Can you work these out from the model? Positions are in its coordinate system, mm. Face numbers are marked on the shaded views. Give positions to 0.01 mm unless a question says otherwise; leave off trailing zeros. Write each loop counter-clockwise with the first axis right and the second up, starting at its lowest first coordinate (ties: lowest second). Pieces come first, ordered by that corner, then holes. Notation, with made-up numbers: (20.5, 27) -> (51.5, 27) arc R29 ccw to (51.5, 64) -> close; hole circle Ø11 at (-35.75, 60). An arc over 180 degrees is marked (long way). Answer as CSV lines item,"result". Start each with the question number.
1. If we section it at D-D on y = -1.65: Write out the boundary of the cut face in (x, z).
2. I need wall thicknesses on line 1 (Y direction, x = 11.5, z = 3.25); line 2 (X direction, y = -0.9, z = 3.2); line 3 (X direction, y = -0.15, z = 2.35). Which ranges of each line are inside material? Lowest first, please. Write a range as [from, to].
3. If we section it at B-B on y = -0.6: Write out the boundary of the cut face in (x, z).
4. If we section it at A-A on z = 3.5: Count the separate pieces of the cut face and the enclosed holes in it, plus the area to 3 significant figures.
5. If we section it at C-C on y = 0.55: Write out the boundary of the cut face in (x, z).
6. If we mould it in two halves opening along Y, with no side actions, what happens to the marked faces 1, 2 and 3? For each: pulls with the +Y half, pulls with the -Y half, needs draft (parallel to the pull), parting line crosses it, or undercut.
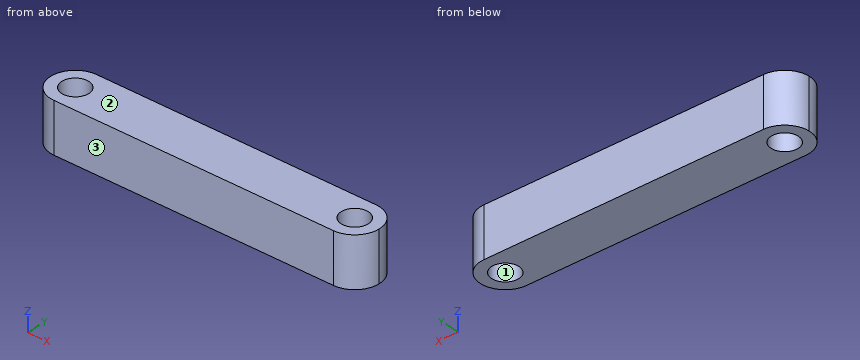
```python
from build123d import *

# Parameters (mm, degrees)
SKETCH_1_W          = 27
SKETCH_1_H          = 4
EXTRUDE_1_DEPTH     = 4
FILLET_1_R          = 2
SKETCH_2_R          = 1.1
CUT_EXTRUDE_1_DEPTH = 13


with BuildPart() as part:
    # 草图1 → 凸台-拉伸1 (new body)
    with BuildSketch(Plane.XY):
        Rectangle(SKETCH_1_W, SKETCH_1_H)
    extrude(amount=EXTRUDE_1_DEPTH)

    # 圆角1
    fillet_1_edges = [part.edges().sort_by_distance(p)[0] for p in [
        (-13.5, -2, 2),
        (-13.5, 2, 2),
        (13.5, -2, 2),
        (13.5, 2, 2),
    ]]
    fillet(fillet_1_edges, radius=FILLET_1_R - 0.0001)  # a hair under: the kernel refuses the full size

    # 草图2 → 切除-拉伸1 (cut)
    with BuildSketch(Plane.XY.offset(4)):
        with Locations((-11.5, 0)):
            Circle(SKETCH_2_R)
        with Locations((11.5, 0)):
            Circle(SKETCH_2_R)
    extrude(amount=-CUT_EXTRUDE_1_DEPTH, mode=Mode.SUBTRACT)


solid = part.part
```
Computed values:
1,outline,"(-12.63, 0) -> (12.63, 0) -> (12.63, 4) -> (-12.63, 4) -> close"
2,line 1,"y = [-2, -1.1], [1.1, 2]"
2,line 2,"x = [-13.29, -12.13], [-10.87, 10.87], [12.13, 13.29]"
2,line 3,"x = [-13.49, -12.59], [-10.41, 10.41], [12.59, 13.49]"
3,outline,"(-13.41, 0) -> (-12.42, 0) -> (-12.42, 4) -> (-13.41, 4) -> close; (-10.58, 0) -> (10.58, 0) -> (10.58, 4) -> (-10.58, 4) -> close; (12.42, 0) -> (13.41, 0) -> (13.41, 4) -> (12.42, 4) -> close"
4,separate pieces,"1"
4,enclosed holes,"2"
4,area,"97.0 mm2"
5,outline,"(-13.42, 0) -> (-12.45, 0) -> (-12.45, 4) -> (-13.42, 4) -> close; (-10.55, 0) -> (10.55, 0) -> (10.55, 4) -> (-10.55, 4) -> close; (12.45, 0) -> (13.42, 0) -> (13.42, 4) -> (12.45, 4) -> close"
6,face 1,"undercut"
6,face 2,"needs draft"
6,face 3,"pulls with the -Y half"
